Geometry: final body of the model. Coordinates: model frame, mm. Face numbers are marked on the shaded views. A direction names the side the tool comes from. Round coordinates to 2 decimals unless told otherwise and drop trailing zeros. Write each loop counter-clockwise with the first axis right and the second up, starting at its lowest first coordinate (ties: lowest second). Pieces come first, ordered by that corner, then holes. Notation, with made-up numbers: (54, 70.25) -> (113, 70.25) arc R19 cw to (113, 107.25) -> close; hole circle Ø4 at (57.25, 85). An arc over 180 degrees is marked (long way). Use one line per item in the form item = value. Start each with the question number.
1. Cut plane C-C, the plane z = -12. Return the cut outline in (x, y).
2. Cut plane B-B, the plane x = 0. Return the cut outline in (y, z), plus the area to 3 significant figures.
3. Reachability of the marked faces 5, 6 and 7 from +Z, -Z, +X, -X, +Y, -Y: full face, straight path, thin tool, end or side. Return the list, or none.
4. Cut plane A-A, the plane y = 0. State how many separate pieces and enclosed holes the cut face has, plus the area to 3 significant figures.
5. Cut plane D-D, the plane y = -8.5. Return the cut outline in (x, z).
6. Draft query along X for the marked faces 1, 2, 3 and 4. Return one class per face: pulls with the +X half, pulls with the -X half, needs draft (parallel to the pull), parting line crosses it, or undercut.
7. Line query: L1, parallel to X at y = -10, z = 23.5; L2, parallel to X at y = 0, z = -26.5; L3, parallel to Y at x = 22, z = -9. Output: solid intervals per line, ascending.
8. Pin query (flat end, axial travel): pin 1 Ø3 at (x, y) = (-17.5, 0.5) entering from +Z; pin 2 Ø14.5 at (y, z) = (-1, 18) entering from +X; pin 3 Ø12 at (x, z) = (15, 19.5) entering from -Y; pin 4 Ø4 at (x, y) = (18.5, 17) entering from -Z. Return the tip coordinate at first contact, or that it passes through.
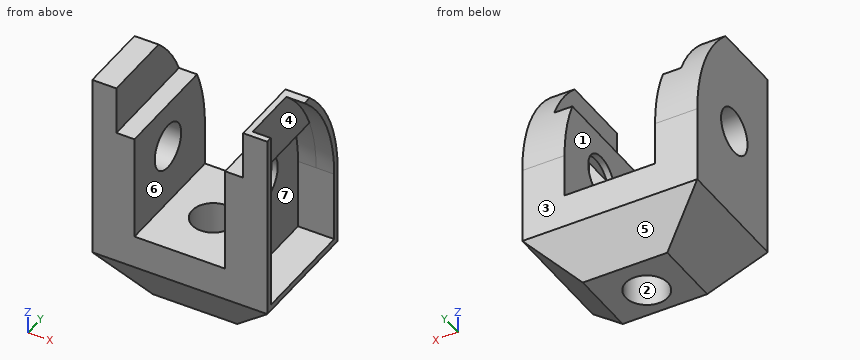
```python
from build123d import *

# Parameters (mm, degrees)
SKETCH1_R           = 7.5
BOSS_EXTRUDE1_DEPTH = 29
CUT_EXTRUDE1_DEPTH  = 68.505555327
SKETCH3_R           = 7
CUT_EXTRUDE2_DEPTH  = 85.917607126
CUT_EXTRUDE3_DEPTH  = 68.505555438
CUT_EXTRUDE4_DEPTH  = 6
CUT_EXTRUDE5_DEPTH  = 6


with BuildPart() as part:
    # Sketch1 → Boss-Extrude1 (new, symmetric)
    with BuildSketch(Plane(origin=(0, 0, 0), x_dir=(0, 0, -1), z_dir=(1, 0, 0))):
        with BuildLine():
            Line((-31, 5), (-31, -19))
            Line((-31, -19), (31, -19))
            Line((31, -19), (46, -10.339745962))
            Line((46, -10.339745962), (46, 12.339745962))
            Line((46, 12.339745962), (31, 21))
            Line((31, 21), (5.66060556, 21))
            ThreePointArc((5.66060556, 21), (-14.33939444, 16.82575695), (-31, 5))
        make_face()
        with Locations(Location((0, 0, 0), (0, 0, 180))):
            Circle(SKETCH1_R, mode=Mode.SUBTRACT)
    extrude(amount=BOSS_EXTRUDE1_DEPTH, both=True)

    # Sketch2 → Cut-Extrude1 (cut, through all)
    with BuildSketch(Plane(origin=(0, 21, 0), x_dir=(1, 0, 0), z_dir=(0, 1, 0))):
        Polygon((-29, 31), (-14, 46), (-29, 46), align=None)
        Polygon((29, 31), (29, 46), (14, 46), align=None)
    extrude(amount=-CUT_EXTRUDE1_DEPTH, mode=Mode.SUBTRACT)

    # Sketch3 → Cut-Extrude2 (cut, through all)
    with BuildSketch(Plane(origin=(0, 0, -46), x_dir=(-1, 0, 0), z_dir=(0, 0, -1))):
        with Locations(Location((0, 0, 0), (0, 0, 90))):
            Circle(SKETCH3_R)
    extrude(amount=-CUT_EXTRUDE2_DEPTH, mode=Mode.SUBTRACT)

    # Sketch4 → Cut-Extrude3 (cut, through all)
    with BuildSketch(Plane(origin=(0, 21, 0), x_dir=(1, 0, 0), z_dir=(0, 1, 0))):
        Polygon((-21, -31), (21, -31), (21, -15), (15, -15), (15, 20), (-15, 20), (-15, -15), (-21, -15), align=None)
    extrude(amount=-CUT_EXTRUDE3_DEPTH, mode=Mode.SUBTRACT)

    # Sketch6 → Cut-Extrude4 (cut)
    with BuildSketch(Plane(origin=(29, 0, 0), x_dir=(0, 0, -1), z_dir=(1, 0, 0))):
        with BuildLine():
            Line((-31, 2.058823529), (-31, -17))
            Line((-31, -17), (29, -17))
            Line((29, -17), (29, 19))
            Line((29, 19), (5.66060556, 19))
            ThreePointArc((5.66060556, 19), (-13.53939444, 14.992726672), (-29.533575778, 3.64))
            Line((-29.533575778, 3.64), (-31, 2.058823529))
        make_face()
    extrude(amount=-CUT_EXTRUDE4_DEPTH, mode=Mode.SUBTRACT)

    # Sketch7 → Cut-Extrude5 (cut)
    with BuildSketch(Plane(origin=(23, 0, 0), x_dir=(0, 0, -1), z_dir=(1, 0, 0))):
        with BuildLine():
            Line((-13, -17), (29, -17))
            Line((29, -17), (29, 19))
            Line((29, 19), (5.66060556, 19))
            ThreePointArc((5.66060556, 19), (-3.858778616, 18.046586751), (-13, 15.224221872))
            Line((-13, 15.224221872), (-13, -17))
        make_face()
    extrude(amount=-CUT_EXTRUDE5_DEPTH, mode=Mode.SUBTRACT)


solid = part.part
```
Outcome:
q1.outline = (-29, -19) -> (-15, -19) -> (-15, 21) -> (-29, 21) -> close; (15, -19) -> (29, -19) -> (29, -17) -> (17, -17) -> (17, 19) -> (29, 19) -> (29, 21) -> (15, 21) -> close
q2.outline = (-19, -31) -> (-10.34, -46) -> (-7, -46) -> (-7, -20) -> (-19, -20) -> close; (7, -46) -> (12.34, -46) -> (21, -31) -> (21, -20) -> (7, -20) -> close
q2.area = 546 mm^2
q3.face_5 = -Z, +X, -X, +Y
q3.face_6 = +Z, +Y, -Y
q3.face_7 = +X
q4.separate_pieces = 4
q4.enclosed_holes = 0
q4.area = 1,300 mm^2
q5.outline = (-29, -31) -> (-14, -46) -> (14, -46) -> (29, -31) -> (29, -29) -> (17, -29) -> (17, 13) -> (23, 13) -> (23, 31) -> (21, 31) -> (21, 15) -> (15, 15) -> (15, -20) -> (-15, -20) -> (-15, 15) -> (-21, 15) -> (-21, 31) -> (-29, 31) -> close
q6.face_1 = undercut
q6.face_2 = undercut
q6.face_3 = needs draft
q6.face_4 = pulls with the +X half
q7.L1 = -29 to -21, 21 to 23
q7.L2 = -29 to -7, 7 to 17
q7.L3 = -19 to -17, 19 to 21
q8.pin_1 = 15
q8.pin_2 = 23
q8.pin_3 = -19
q8.pin_4 = -41.39
